```python
from build123d import *

# Parameters (mm, degrees)
SKETCH1_W           = 150
SKETCH1_H           = 3
BOSS_EXTRUDE1_DEPTH = 121
SKETCH3_W           = 21.1
SKETCH3_H           = 64.5
CUT_EXTRUDE1_DEPTH  = 1
SKETCH4_W           = 21.1
SKETCH4_H           = 64.5
CUT_EXTRUDE2_DEPTH  = 1
SKETCH6_W           = 6.5
SKETCH6_H           = 4.8
BOSS_EXTRUDE5_DEPTH = 3
SKETCH9_W           = 6.5
SKETCH9_H           = 5.03681905
BOSS_EXTRUDE7_DEPTH = 3
SKETCH10_W          = 150
SKETCH10_H          = 25
BOSS_EXTRUDE8_DEPTH = 2.5


with BuildPart() as part:
    # Sketch1 → Boss-Extrude1 (new body)
    with BuildSketch(Plane.XY):
        with Locations((75, 1.5)):
            Rectangle(SKETCH1_W, SKETCH1_H)
    extrude(amount=BOSS_EXTRUDE1_DEPTH)

    # Sketch3 → Cut-Extrude1 (cut)
    with BuildSketch(Plane(origin=(0, 3, 0), x_dir=(1, 0, 0), z_dir=(0, 1, 0))):
        with Locations((10.55, -86.824661278)):
            Rectangle(SKETCH3_W, SKETCH3_H)
    extrude(amount=-CUT_EXTRUDE1_DEPTH, mode=Mode.SUBTRACT)

    # Sketch4 → Cut-Extrude2 (cut)
    with BuildSketch(Plane(origin=(0, 3, 0), x_dir=(1, 0, 0), z_dir=(0, 1, 0))):
        with Locations((139.45, -87.298299378)):
            Rectangle(SKETCH4_W, SKETCH4_H)
    extrude(amount=-CUT_EXTRUDE2_DEPTH, mode=Mode.SUBTRACT)

    # Sketch6 → Boss-Extrude5 (add)
    with BuildSketch(Plane(origin=(0, 0, 0), x_dir=(1, 0, 0), z_dir=(0, 1, 0))):
        with Locations((-3.25, -24.887330639)):
            Rectangle(SKETCH6_W, SKETCH6_H)
    extrude(amount=BOSS_EXTRUDE5_DEPTH)

    # Sketch9 → Boss-Extrude7 (add)
    with BuildSketch(Plane(origin=(0, 3, 0), x_dir=(1, 0, 0), z_dir=(0, 1, 0))):
        with Locations((153.25, -25.005740164)):
            Rectangle(SKETCH9_W, SKETCH9_H)
    extrude(amount=-BOSS_EXTRUDE7_DEPTH)

    # Sketch10 → Boss-Extrude8 (add)
    with BuildSketch(Plane(origin=(0, 0, 0), x_dir=(-1, 0, 0), z_dir=(0, 0, -1))):
        with Locations((-75, 15.5)):
            Rectangle(SKETCH10_W, SKETCH10_H)
    extrude(amount=-BOSS_EXTRUDE8_DEPTH)


solid = part.part
```
Here's how the part is built. I have some questions about the finished solid (model axes, mm). A direction names the side the tool comes from. Give positions to 0.01 mm unless a question says otherwise; leave off trailing zeros. Loops run counter-clockwise (first coordinate to the right, second up) from the corner with the lowest first, then second, coordinate; pieces in that order, holes last. Notation, with made-up numbers: M 2,-21 L 56,-21 A25 ccw 56,-9 Z; hole C 14,-32 d9. An arc over 180 degrees is marked long. Return JSON: item names as keys, results as strings.
Item 1: Imagine slicing it at C-C on y = 15.25. List the corners of the cut face in (x, z) for me.
A:
{"outline": "M 0,0 L 150,0 L 150,2.5 L 0,2.5 Z"}
Item 2: Imagine slicing it at B-B on x = 47.5. List the corners of the cut face in (y, z) for me.
A:
{"outline": "M 0,0 L 28,0 L 28,2.5 L 3,2.5 L 3,121 L 0,121 Z"}
Item 3: Imagine slicing it at D-D on z = 41.5. List the corners of the cut face in (x, y) for me.
A:
{"outline": "M 0,0 L 150,0 L 150,3 L 0,3 Z"}
Item 4: On a 3-axis mill with a long thin cutter (end or side, diameter ignored), from which of +Z, -Z, +X, -X, +Y, -Y can I reach the whole of each face in a straight line? I mean faces 5 (the flat face through (74, 0, 60)), 6 (the flat face through (74, 3, 61)), 7 (the flat face through (150, 8, 2)). Say none if no direction works.
A:
{"face 5": "+Z, -Z, +X, -X, -Y", "face 6": "+Z, +X, -X, +Y", "face 7": "-Z, +X, +Y, -Y"}
Item 5: Thinking about a two-plate mould opening in Z: for faces 1 (the flat face through (139, 2, 87)), 2 (the flat face through (10, 2, 86)), 3 (the flat face through (76, 14, 0)), 4 (the flat face through (0, 8, 2)), which applies, released by +Z, released by -Z, zero draft, split by the parting line, or undercut?
A:
{"face 1": "undercut", "face 2": "undercut", "face 3": "released by -Z", "face 4": "zero draft"}
Item 6: Imagine slicing it at A-A on z = 63. List the corners of the cut face in (x, y) for me.
A:
{"outline": "M 0,0 L 150,0 L 150,2 L 128.9,2 L 128.9,3 L 21.1,3 L 21.1,2 L 0,2 Z"}
Item 7: I'm going to push flat-ended pins straight in: pin 1 Ø1 at (x, z) = (49, 50) entering from -Y; pin 2 Ø3 at (x, y) = (115, 18.5) entering from +Z; pin 3 Ø6.5 at (x, z) = (5.5, 89.5) entering from +Y; pin 4 Ø1.5 at (y, z) = (2, 73.5) entering from +X. Where does each tip first touch, or does it pass through?
A:
{"pin 1": "stops at y = 0", "pin 2": "stops at z = 2.5", "pin 3": "stops at y = 2", "pin 4": "stops at x = 150"}
Item 8: Please list where these lines run through material, in increasing order: line 1 (Z direction, x = 147, y = 2.25); line 2 (Y direction, x = 142, z = 41.5); line 3 (Y direction, x = 17, z = 104.5).
A:
{"line 1": "z = 0 to 55.05, 119.55 to 121", "line 2": "y = 0 to 3", "line 3": "y = 0 to 2"}
